Can you work these out from the model? Positions are in its coordinate system, mm. Face numbers are marked on the shaded views. A direction names the side the tool comes from. Coordinates: 2 decimals unless noted, no trailing zeros. Order: outer loops, then holes, each group sorted by start corner. A loop starts at its lowest first (then second) coordinate and runs counter-clockwise, first axis right, second up. Notation, with made-up numbers: (-8, 59) -> (38, 59) arc R20 cw to (38, 64) -> close; hole circle Ø7 at (78, -27.75). An arc over 180 degrees is marked (long way). Answer in a Markdown table with one row per item.
```python
from build123d import *

# Parameters (mm, degrees)
BOSS_EXTRUDE1_DEPTH = 4
SKETCH2_R           = 0.79375
CUT_EXTRUDE1_DEPTH  = 4


with BuildPart() as part:
    # Sketch1 → Boss-Extrude1 (new body)
    with BuildSketch(Plane.XY):
        Polygon((-19.05, 32.916114), (31.75, 32.916114), (31.75, 31.931727843), (27.640915, 30.869046207), (27.640915, 28.978433793), (31.75, 27.915752157), (31.75, 25.946979843), (27.640915, 24.884298207), (27.640915, 22.993685793), (31.75, 21.931004157), (31.75, 19.962231843), (27.640915, 18.899550207), (27.640915, 17.008937793), (31.75, 15.946256157), (31.75, 13.977483843), (27.640915, 12.914802207), (27.640915, 11.024189793), (31.75, 9.961508157), (31.75, 7.992735843), (27.640915, 6.930054207), (27.640915, 5.039441793), (31.75, 3.976760157), (31.75, 2.007987843), (27.640915, 0.945306207), (27.640915, 0), (-14.940915, 0), (-14.940915, 0.945306207), (-19.05, 2.007987843), (-19.05, 3.976760157), (-14.940915, 5.039441793), (-14.940915, 6.930054207), (-19.05, 7.992735843), (-19.05, 9.961508157), (-14.940915, 11.024189793), (-14.940915, 12.914802207), (-19.05, 13.977483843), (-19.05, 15.946256157), (-14.940915, 17.008937793), (-14.940915, 18.899550207), (-19.05, 19.962231843), (-19.05, 21.931004157), (-14.940915, 22.993685793), (-14.940915, 24.884298207), (-19.05, 25.946979843), (-19.05, 27.915752157), (-14.940915, 28.978433793), (-14.940915, 30.869046207), (-19.05, 31.931727843), align=None)
    extrude(amount=BOSS_EXTRUDE1_DEPTH)

    # Sketch2 → Cut-Extrude1 (cut)
    with BuildSketch(Plane.XY.offset(4)):
        with Locations((-1.27, 17.676114)):
            Circle(SKETCH2_R)
        with Locations((24.13, 17.676114)):
            Circle(SKETCH2_R)
        with Locations((24.13, 4.976114)):
            Circle(SKETCH2_R)
        with Locations((-1.27, 4.976114)):
            Circle(SKETCH2_R)
    extrude(amount=-CUT_EXTRUDE1_DEPTH, mode=Mode.SUBTRACT)


solid = part.part
```
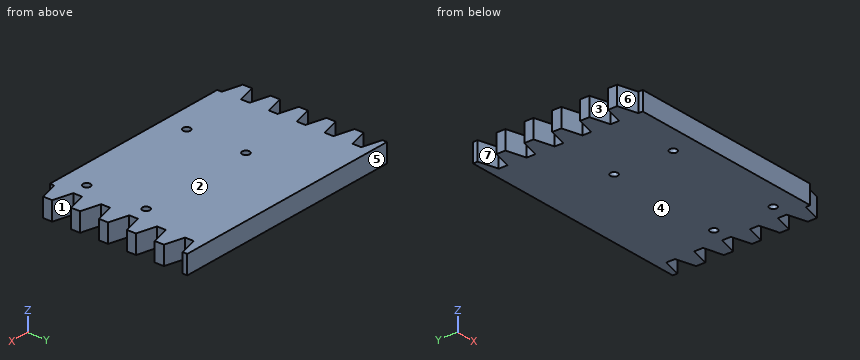
(1) Will these pins go through, and if not, where does the flat tip stop? pin 1 Ø0.9 at (y, z) = (12, 2) entering from -X; pin 2 Ø0.9 at (y, z) = (30, 2) entering from +X.
Response values:
| item | result |
|---|---|
| pin 1 | x = -14.94 |
| pin 2 | x = 27.64 |
(2) I need wall thicknesses on line 1 (Y direction, x = 24.13, z = 1.2); line 2 (X direction, y = 29, z = 0.5); line 3 (Y direction, x = -1.5, z = 2.1). Which ranges of each line are inside material? Lowest first, please. Write a range as [from, to].
Response values:
| item | result |
|---|---|
| line 1 | [0, 4.18], [5.77, 16.88], [18.47, 32.92] |
| line 2 | [-14.94, 27.64] |
| line 3 | [0, 4.22], [5.74, 16.92], [18.44, 32.92] |
(3) Suppose I cut it at B-B (y = 29.5). Please give me the cut outline in (x, z).
Response values:
| item | result |
|---|---|
| outline | (-14.94, 0) -> (27.64, 0) -> (27.64, 4) -> (-14.94, 4) -> close |
(4) On a 3-axis mill with a long thin cutter (end or side, diameter ignored), from which of +Z, -Z, +X, -X, +Y, -Y can I reach the whole of each face in a straight line? I mean the marked faces 1, 2 and 3. Say none if no direction works.
Response values:
| item | result |
|---|---|
| face 1 | +Z, -Z, +X |
| face 2 | +Z, +X, -X, +Y, -Y |
| face 3 | +Z, -Z, -X |
(5) Suppose I cut it at C-C (y = 10.5). Please give me the cut outline in (x, z), and give its area (3 significant figures).
Response values:
| item | result |
|---|---|
| outline | (-16.97, 0) -> (29.67, 0) -> (29.67, 4) -> (-16.97, 4) -> close |
| area | 187 mm2 |
(6) We'd pull the mould along Y, two halves only. Please class the marked faces 4, 5, 6 and 7: +Y half, -Y half, draft (parallel to the pull), parting line (faces both ways), or undercut.
Response values:
| item | result |
|---|---|
| face 4 | draft |
| face 5 | +Y half |
| face 6 | -Y half |
| face 7 | undercut |
(7) Suppose I cut it at A-A (x = -1.27). Please give me the cut outline in (y, z), and give its area (3 significant figures).
Response values:
| item | result |
|---|---|
| outline | (0, 0) -> (4.18, 0) -> (4.18, 4) -> (0, 4) -> close; (5.77, 0) -> (16.88, 0) -> (16.88, 4) -> (5.77, 4) -> close; (18.47, 0) -> (32.92, 0) -> (32.92, 4) -> (18.47, 4) -> close |
| area | 119 mm2 |
